```python
from build123d import *

# Parameters (mm, degrees)
MODEL_R                 = 1.5
MODEL_R_2               = 4.5
SALIENTE_EXTRUIR1_DEPTH = 3


with BuildPart() as part:
    # Model → Saliente-Extruir1 (new body)
    with BuildSketch(Plane.XY):
        with BuildLine():
            Line((206.945286968, 204.077019993), (199.609852846, 238.514519993))
            ThreePointArc((199.609852846, 238.514519993), (215.747807914, 258.452019993), (231.885762981, 238.514519993))
            Line((231.885762981, 238.514519993), (224.550328859, 204.077019993))
            ThreePointArc((224.550328859, 204.077019993), (215.747807914, 196.952019993), (206.945286968, 204.077019993))
        make_face()
        with Locations((215.747807914, 241.952019993)):
            Circle(MODEL_R, mode=Mode.SUBTRACT)
        with Locations((215.747807914, 232.952019993)):
            Circle(MODEL_R, mode=Mode.SUBTRACT)
        with Locations((215.747807914, 250.952019993)):
            Circle(MODEL_R, mode=Mode.SUBTRACT)
        with Locations((215.747807914, 205.952019993)):
            Circle(MODEL_R_2, mode=Mode.SUBTRACT)
        with BuildLine():
            Line((223.122807913, 245.202019993), (221.372807913, 245.202019993))
            ThreePointArc((221.372807913, 245.202019993), (220.842477828, 244.982350079), (220.622807913, 244.452019993))
            Line((220.622807913, 244.452019993), (220.622807913, 239.452019993))
            ThreePointArc((220.622807913, 239.452019993), (220.842477828, 238.921689907), (221.372807913, 238.702019993))
            Line((221.372807913, 238.702019993), (223.122807913, 238.702019993))
            ThreePointArc((223.122807913, 238.702019993), (223.653137999, 238.921689907), (223.872807913, 239.452019993))
            Line((223.872807913, 239.452019993), (223.872807913, 244.452019993))
            ThreePointArc((223.872807913, 244.452019993), (223.653137999, 244.982350079), (223.122807913, 245.202019993))
        make_face(mode=Mode.SUBTRACT)
        with BuildLine():
            Line((208.372807913, 245.202019993), (210.122807913, 245.202019993))
            ThreePointArc((210.122807913, 245.202019993), (210.653137999, 244.982350079), (210.872807913, 244.452019993))
            Line((210.872807913, 244.452019993), (210.872807913, 239.452019993))
            ThreePointArc((210.872807913, 239.452019993), (210.653137999, 238.921689907), (210.122807913, 238.702019993))
            Line((210.122807913, 238.702019993), (208.372807913, 238.702019993))
            ThreePointArc((208.372807913, 238.702019993), (207.842477828, 238.921689907), (207.622807913, 239.452019993))
            Line((207.622807913, 239.452019993), (207.622807913, 244.452019993))
            ThreePointArc((207.622807913, 244.452019993), (207.842477828, 244.982350079), (208.372807913, 245.202019993))
        make_face(mode=Mode.SUBTRACT)
    extrude(amount=SALIENTE_EXTRUIR1_DEPTH)


solid = part.part
```
Geometry: final body of the model. Coordinates: model frame, mm. A direction names the side the tool comes from. Coordinates: 2 decimals unless noted, no trailing zeros. Loops run counter-clockwise (first coordinate to the right, second up) from the corner with the lowest first, then second, coordinate; pieces in that order, holes last. Notation, with made-up numbers: (-1.75, -28.5) -> (30.25, -28.5) arc R27 ccw to (30.25, 1.5) -> close; hole circle Ø3 at (38, 19.25). An arc over 180 degrees is marked (long way). Use a Markdown table: item, result. Add a question column.
(1) Section query A-A, the plane x = 212. Return loops of the section in (y, z), plus the area to 3 significant figures.
(2) Section query C-C, the plane y = 253.5. Return loops of the section in (x, z).
(3) Section query B-B, the plane z = 0.45. Return loops of the section in (x, y), plus the area to 3 significant figures.
(4) Mould query, pull axis X, two halves, no side actions, for faces 3 (the flat face through (228.27, 221.54, 1.48)), 4 (the flat face through (203.33, 221.05, 1.48)), 5 (the flat face through (209, 238.702, 1)). Classes: pulls with the +X half, pulls with the -X half, needs draft (parallel to the pull), parting line crosses it, or undercut.
(5) Line query: line 1 along Y through (x, z) = (215, 1.05); line 2 along X through (y, z) = (239, 1.4); line 3 along Y through (x, z) = (214.5, 1.6). Output: solid intervals per line, ascending.
(6) Access query for faces 1 (the cylindrical face through (215.919, 196.954, 1.479)), 2 (the flat face through (222, 238.702, 1)). Directions: +Z, -Z, +X, -X, +Y, -Y. A direction counts if a zero-diameter tool reaches every point of the face in a straight line with its end or side. Return the directions, or none.
(7) Pin query (flat end, axial travel): pin 1 Ø0.9 at (y, z) = (243, 2) entering from +X; pin 2 Ø4 at (x, y) = (215.75, 232.95) entering from -Z; pin 3 Ø0.5 at (x, z) = (209, 1) entering from +Y; pin 4 Ø1.4 at (x, z) = (222, 1.5) entering from -Y. Return the tip coordinate at first contact, or that it passes through.
(8) Section query D-D, the plane x = 201. Return loops of the section in (y, z), plus the area to 3 significant figures.
Answer:
| question | item | result |
|---|---|---|
| 1 | outline | (197.77, 0) -> (203.46, 0) -> (203.46, 3) -> (197.77, 3) -> close; (208.44, 0) -> (258.02, 0) -> (258.02, 3) -> (208.44, 3) -> close |
| 1 | area | 166 mm^2 |
| 2 | outline | (203.96, 0) -> (227.53, 0) -> (227.53, 3) -> (203.96, 3) -> close |
| 3 | outline | (199.61, 238.51) -> (206.95, 204.08) arc R9 ccw to (224.55, 204.08) -> (231.89, 238.51) arc R16.5 ccw (long way) to start; hole (207.62, 239.45) arc R0.75 ccw to (208.37, 238.7) -> (210.12, 238.7) arc R0.75 ccw to (210.87, 239.45) -> (210.87, 244.45) arc R0.75 ccw to (210.12, 245.2) -> (208.37, 245.2) arc R0.75 ccw to (207.62, 244.45) -> close; hole circle Ø9 at (215.75, 205.95); hole circle Ø3 at (215.75, 232.95); hole circle Ø3 at (215.75, 241.95); hole circle Ø3 at (215.75, 250.95); hole (220.62, 239.45) arc R0.75 ccw to (221.37, 238.7) -> (223.12, 238.7) arc R0.75 ccw to (223.87, 239.45) -> (223.87, 244.45) arc R0.75 ccw to (223.12, 245.2) -> (221.37, 245.2) arc R0.75 ccw to (220.62, 244.45) -> close |
| 3 | area | 1,370 mm^2 |
| 4 | face 3 | pulls with the +X half |
| 4 | face 4 | pulls with the -X half |
| 4 | face 5 | undercut |
| 5 | line 1 | y = 196.98 to 201.51, 210.39 to 231.65, 234.25 to 240.65, 243.25 to 249.65, 252.25 to 258.44 |
| 5 | line 2 | x = 199.51 to 207.77, 210.72 to 220.77, 223.72 to 231.98 |
| 5 | line 3 | y = 197.04 to 201.63, 210.28 to 232.12, 233.78 to 241.12, 242.78 to 250.12, 251.78 to 258.4 |
| 6 | face 1 | +Z, -Z, -Y |
| 6 | face 2 | +Z, -Z |
| 7 | pin 1 | stops at x = 232.24 |
| 7 | pin 2 | stops at z = 0 |
| 7 | pin 3 | stops at y = 257.12 |
| 7 | pin 4 | stops at y = 198.87 |
| 8 | outline | (231.99, 0) -> (249.35, 0) -> (249.35, 3) -> (231.99, 3) -> close |
| 8 | area | 52.1 mm^2 |
